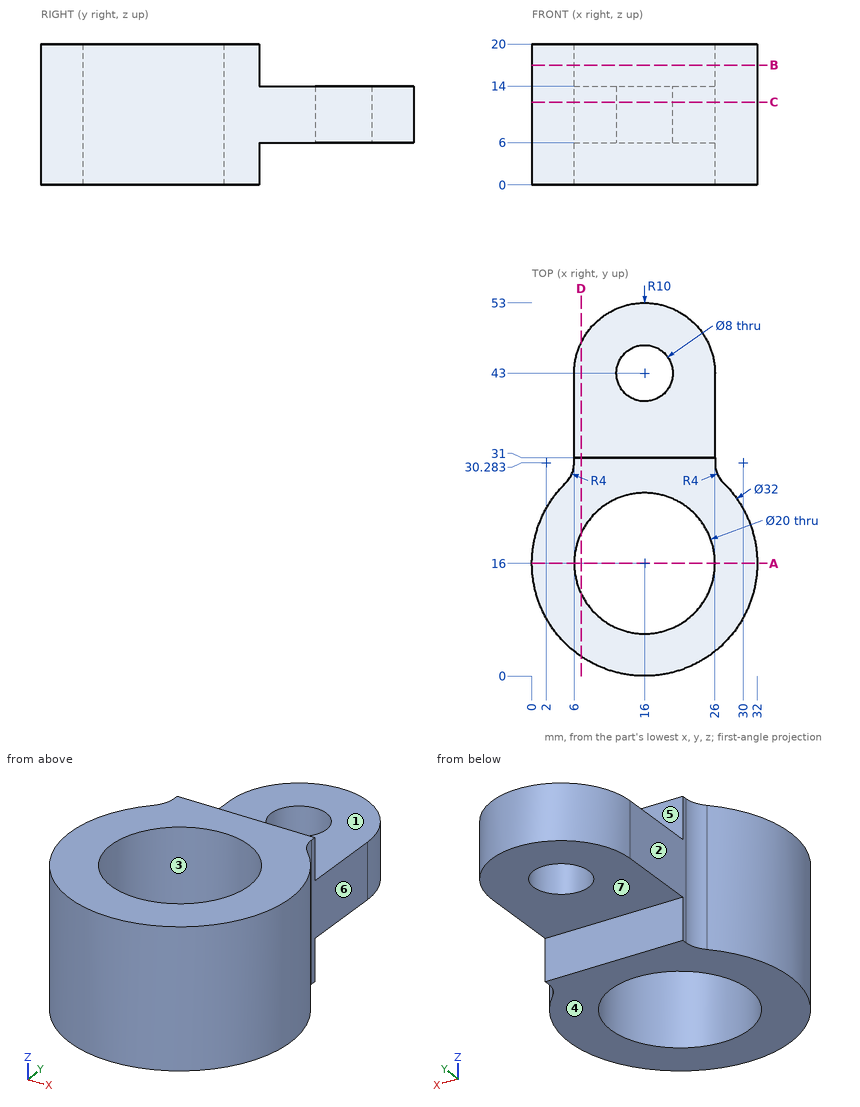
Part print with two shaded views. Sizes in mm from the minimum x, y, z corner. A direction names the side the tool comes from. Round coordinates to 2 decimals unless told otherwise and drop trailing zeros. Write each loop counter-clockwise with the first axis right and the second up, starting at its lowest first coordinate (ties: lowest second). Pieces come first, ordered by that corner, then holes. Notation, with made-up numbers: (-24, -1.75) - (9, -1.75) arc R25 cw to (9, 13.25) - close; hole circle Ø6 at (-31.75, 40). An arc over 180 degrees is marked (long way). Use CSV: the item, a comma, the result in double quotes.
Item 1: Slice it at B-B, the plane z = 17. Write the cut outline in (x, y), then the cut area to 3 significant figures.
Results list:
outline,"(4.8, 27.43) arc R16 ccw (long way) to (27.2, 27.43) arc R4 cw to (26, 30.28) - (26, 31) - (6, 31) - (6, 30.28) arc R4 cw to start; hole circle Ø20 at (16, 16)"
area,"493 mm²"
Item 2: Tool access for the marked faces 4, 5, 6 and 7: list every direction of +Z, -Z, +X, -X, +Y, -Y with a clear straight run to the whole face (end or side of a thin tool).
Results list:
face 4,"-Z, +X, -X, +Y, -Y"
face 5,"+Z, +X, -X, +Y"
face 6,"+Z, -Z, +X, +Y"
face 7,"-Z, +X, -X, +Y"
Item 3: Flat gauge pins, fed straight in: P1, Ø8, axis at x = 6, z = 11, coming from the -Y side; P2, Ø12, axis at y = 9, z = 16.5, coming from the -X side; P3, Ø5, axis at x = 6, z = 17, coming from the -Y side; P4, Ø16, axis at x = 16, y = 16, coming from the -Z side. Where does each tip first touch, or does it go through?
Results list:
P1,"stops at y = 1.17"
P2,"stops at x = 0.03"
P3,"stops at y = 1.87"
P4,"passes through"
Item 4: Slice it at A-A, the plane y = 16. Write the cut outline in (x, z), then the cut area to 3 significant figures.
Results list:
outline,"(0, 0) - (6, 0) - (6, 20) - (0, 20) - close; (26, 0) - (32, 0) - (32, 20) - (26, 20) - close"
area,"240 mm²"
Item 5: Slice it at D-D, the plane x = 7. Write the cut outline in (y, z), then the cut area to 3 significant figures.
Results list:
outline,"(2.77, 0) - (11.64, 0) - (11.64, 20) - (2.77, 20) - close; (20.36, 0) - (31, 0) - (31, 6) - (47.36, 6) - (47.36, 14) - (31, 14) - (31, 20) - (20.36, 20) - close"
area,"521 mm²"
Item 6: Pull direction X, two halves, no side cores. Call the marked faces 1, 2 and 3: pulls with the +X half, pulls with the -X half, needs draft (parallel to the pull), parting line crosses it, or undercut.
Results list:
face 1,"needs draft"
face 2,"pulls with the -X half"
face 3,"undercut"
Item 7: Wall check: L1, parallel to X at y = 16.5, z = 2.5; L2, parallel to Y at x = 18.5, z = 10; L3, parallel to X at y = 43, z = 12. Give the ranges that are in metal, low to high.
Results list:
L1,"x = 0.01 to 6.01, 25.99 to 31.99"
L2,"y = 0.2 to 6.32, 25.68 to 39.88, 46.12 to 52.68"
L3,"x = 6 to 12, 20 to 26"
Item 8: Slice it at C-C, the plane z = 11.75. Write the cut outline in (x, y), then the cut area to 3 significant figures.
Results list:
outline,"(4.8, 27.43) arc R16 ccw (long way) to (27.2, 27.43) arc R4 cw to (26, 30.28) - (26, 43) arc R10 ccw to (6, 43) - (6, 30.28) arc R4 cw to start; hole circle Ø20 at (16, 16); hole circle Ø8 at (16, 43)"
area,"840 mm²"
